from build123d import *

# Parameters (mm, degrees)
SKETCH1_W           = 54.61
SKETCH1_H           = 47.244
SKETCH1_W_2         = 41.91
SKETCH1_H_2         = 21.844
BOSS_EXTRUDE1_DEPTH = 5.08
SKETCH2_R           = 0.93599
SKETCH2_R_2         = 0.635
CUT_EXTRUDE1_DEPTH  = 73.388217522
BOSS_EXTRUDE3_DEPTH = 5.08
SKETCH9_W           = 76.2
SKETCH9_H           = 3.175
CUT_EXTRUDE2_DEPTH  = 0.635


with BuildPart() as part:
    # Sketch1 → Boss-Extrude1 (new body)
    with BuildSketch(Plane.XY):
        with Locations((27.305, 23.622)):
            Rectangle(SKETCH1_W, SKETCH1_H)
        with Locations((27.305, 23.622)):
            Rectangle(SKETCH1_W_2, SKETCH1_H_2, mode=Mode.SUBTRACT)
    extrude(amount=BOSS_EXTRUDE1_DEPTH)

    # Sketch2 → Cut-Extrude1 (cut, through all)
    with BuildSketch(Plane.XY.offset(5.08)):
        with Locations((2.80543, 28.62199)):
            Circle(SKETCH2_R)
        with Locations((2.80543, 18.62201)):
            Circle(SKETCH2_R)
        with Locations((51.80457, 28.62199)):
            Circle(SKETCH2_R)
        with Locations((51.80457, 18.62201)):
            Circle(SKETCH2_R)
        with Locations((25.17521, 5.08)):
            Circle(SKETCH2_R_2)
        with Locations((29.43479, 5.08)):
            Circle(SKETCH2_R_2)
        with Locations((29.43479, 42.164)):
            Circle(SKETCH2_R_2)
        with Locations((25.17521, 42.164)):
            Circle(SKETCH2_R_2)
    extrude(amount=-CUT_EXTRUDE1_DEPTH, mode=Mode.SUBTRACT)

    # Sketch8 → Boss-Extrude3 (add)
    with BuildSketch(Plane.XY.offset(5.08)):
        Polygon((0, 0), (-13.335, 0), (-13.335, -12.7), (67.945, -12.7), (67.945, 0), (54.61, 0), align=None)
    extrude(amount=-BOSS_EXTRUDE3_DEPTH)

    # Sketch9 → Cut-Extrude2 (cut)
    with BuildSketch(Plane.XY.offset(5.08)):
        with Locations((27.305, -6.35)):
            Rectangle(SKETCH9_W, SKETCH9_H)
    extrude(amount=-CUT_EXTRUDE2_DEPTH, mode=Mode.SUBTRACT)


solid = part.part
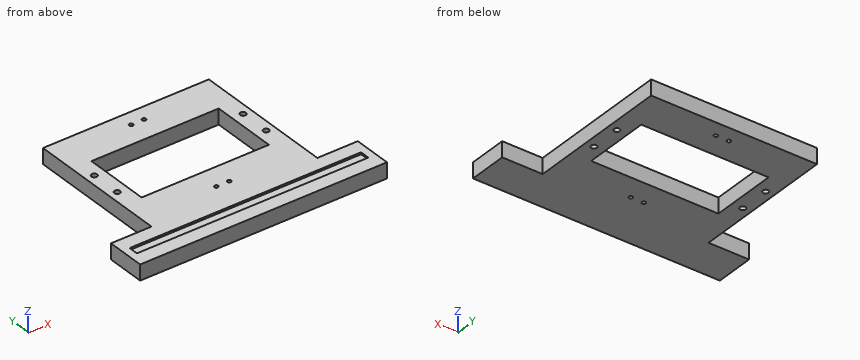
Could you check a few things on this model? Use its own coordinates, in mm. Coordinates: 2 decimals unless noted, no trailing zeros. Order: outer loops, then holes, each group sorted by start corner. A loop starts at its lowest first (then second) coordinate and runs counter-clockwise, first axis right, second up. Notation, with made-up numbers: (-10, -33) - (7, -33) arc R27 ccw to (7, -3) - close; hole circle Ø4 at (8.5, -19.5). An arc over 180 degrees is marked (long way). Answer in a Markdown table with one row per item. Add a question column.
(1) If we section it at B-B, the plane x = 14: Please give me the cut outline in (y, z) (1 decimal), then the cut area to 3 significant figures.
(2) If we section it at C-C, the plane x = 63.5: Please give me the cut outline in (y, z) (1 decimal).
(3) I need wall thicknesses on L1, parallel to Y at x = 10.5, z = 2.85; L2, parallel to X at y = 28.5, z = 1.3; L3, parallel to Y at x = -6.5, z = 4.85. Which ranges of each line are inside material? Lowest first, please.
(4) If we section it at D-D, the plane z = 2.2: State how many separate pieces and enclosed holes the cut face has, then the cut area to 3 significant figures.
(5) Will these pins go through, and if not, where does the flat tip stop? pin 1 (1.6 mm diameter, centred on x = 14, y = -7, fed in from +Z) (3 decimals); pin 2 (1.5 mm diameter, centred on y = 21, z = 3.5, fed in from -X).
(6) If we section it at A-A, the plane y = 15.5: Please give me the cut outline in (x, z), then the cut area to 3 significant figures.
Results are:
| question | item | result |
|---|---|---|
| 1 | outline | (-12.7, 0) - (12.7, 0) - (12.7, 5.1) - (-4.8, 5.1) - (-4.8, 4.4) - (-7.9, 4.4) - (-7.9, 5.1) - (-12.7, 5.1) - close; (34.5, 0) - (47.2, 0) - (47.2, 5.1) - (34.5, 5.1) - close |
| 1 | area | 192 mm2 |
| 2 | outline | (-12.7, 0) - (0, 0) - (0, 5.1) - (-4.8, 5.1) - (-4.8, 4.4) - (-7.9, 4.4) - (-7.9, 5.1) - (-12.7, 5.1) - close |
| 3 | L1 | y = -12.7 to 12.7, 34.54 to 47.24 |
| 3 | L2 | x = 0 to 1.88, 3.73 to 6.35, 48.26 to 50.88, 52.73 to 54.61 |
| 3 | L3 | y = -12.7 to -7.94, -4.76 to 0 |
| 4 | separate pieces | 1 |
| 4 | enclosed holes | 9 |
| 4 | area | 2,680 mm2 |
| 5 | pin 1 | stops at z = 4.445 |
| 5 | pin 2 | stops at x = 0 |
| 6 | outline | (0, 0) - (6.35, 0) - (6.35, 5.08) - (0, 5.08) - close; (48.26, 0) - (54.61, 0) - (54.61, 5.08) - (48.26, 5.08) - close |
| 6 | area | 64.5 mm2 |
